Read the model definition and answer for the solid it produces. Units are mm, in the model's axes. A direction names the side the tool comes from. Coordinates: 2 decimals unless noted, no trailing zeros. Loops run counter-clockwise (first coordinate to the right, second up) from the corner with the lowest first, then second, coordinate; pieces in that order, holes last. Notation, with made-up numbers: M -37,46 L -8,46 A25 ccw -8,58 Z; hole C 29,71.5 d10. An arc over 180 degrees is marked long. One line per item, written item: value. Start each with the question number.
```python
from build123d import *

# Parameters (mm, degrees)
SKETCH1_W           = 93.8
SKETCH1_H           = 32.4
BOSS_EXTRUDE1_DEPTH = 2
SKETCH3_W           = 93.8
SKETCH3_H           = 64.8
SKETCH3_W_2         = 91.4
SKETCH3_H_2         = 62.4
SKETCH3_W_3         = 86.6
SKETCH3_H_3         = 57.6
SKETCH3_W_4         = 83.8
SKETCH3_H_4         = 54.8
BOSS_EXTRUDE2_DEPTH = 4
FILLET6_R           = 2
FILLET8_START       = -66
FILLET8_DEPTH       = 67
FILLET9_R           = 2
FILLET10_R          = 2


with BuildPart() as part:
    # Sketch1 → Boss-Extrude1 (new body)
    with BuildSketch(Plane(origin=(0, 0, 0), x_dir=(1, 0, 0), z_dir=(0, 1, 0))):
        with Locations((46.9, 48.6)):
            Rectangle(SKETCH1_W, SKETCH1_H)
        Polygon((93.8, 32.4), (0, 32.4), (0, 0), (42.9, 0), (50.9, 0), (93.8, 0), align=None)
    extrude(amount=BOSS_EXTRUDE1_DEPTH)

    # Sketch3 → Boss-Extrude2 (add)
    # profile 1 of 2: a face of its own
    with BuildSketch(Plane.XZ):
        with Locations((46.9, -32.4)):
            Rectangle(SKETCH3_W, SKETCH3_H)
        with Locations((46.9, -32.4)):
            Rectangle(SKETCH3_W_2, SKETCH3_H_2, mode=Mode.SUBTRACT)
    # profile 2 of 2: a face of its own
    with BuildSketch(Plane.XZ):
        with Locations((46.9, -32.4)):
            Rectangle(SKETCH3_W_3, SKETCH3_H_3)
        with Locations((46.9, -32.4)):
            Rectangle(SKETCH3_W_4, SKETCH3_H_4, mode=Mode.SUBTRACT)
    extrude(amount=BOSS_EXTRUDE2_DEPTH)

    # Fillet6
    fillet6_edges = [part.edges().sort_by_distance(p)[0] for p in [
        (0, -1, -64.8),
        (93.8, -1, -64.8),
        (93.8, -1, 0),
        (0, -1, 0),
    ]]
    fillet(fillet6_edges, radius=FILLET6_R)

    # Fillet8: read off the stored shape, not the designer's step
    # Fillet8 outline → Fillet8 (cut)
    with BuildSketch(Plane.XY.offset(FILLET8_START)):
        with BuildLine():
            add(Edge.make_bspline(
                [(0, -1), (0, 2), (4, 2)],
                knots=[0, 0, 0, 1, 1, 1], degree=2, weights=[1, 0.707106781, 1]))
            Line((4, 2), (0, 2))
            Line((0, 2), (0, -1))
        make_face()
        with BuildLine():
            add(Edge.make_bspline(
                [(93.8, -1), (93.8, 2), (89.8, 2)],
                knots=[0, 0, 0, 1, 1, 1], degree=2, weights=[1, 0.707106781, 1]))
            Line((93.8, -1), (93.8, 2))
            Line((93.8, 2), (89.8, 2))
        make_face()
    extrude(amount=FILLET8_DEPTH, mode=Mode.SUBTRACT)

    # Fillet9
    fillet9_edges = [part.edges().sort_by_distance(p)[0] for p in [
        (5, 0, -32.4),
        (46.9, 0, -5),
        (88.8, 0, -32.4),
        (46.9, 0, -59.8),
    ]]
    fillet(fillet9_edges, radius=FILLET9_R)

    # Fillet10
    fillet10_edges = [part.edges().sort_by_distance(p)[0] for p in [
        (92.6, -2, -1.2),
    ]]
    fillet(fillet10_edges, radius=FILLET10_R)


solid = part.part
```
1) A flat-ended cylindrical pin translates along its axis: pin 1 (18.5 mm diameter, centred on x = 69, z = -23, fed in from -Y). Find the tip coordinate at first contact, or state that the pin passes through.
2) A tool of negligible diameter and unlimited length cuts with its end or side. For faces 1 (the face through (47, -4, -1)), 2 (the face through (92.6, -2, -34)), from which of +Z, -Z, +X, -X, +Y, -Y can it reach the whole face along a straight path? Write none if from no direction.
3) Section A-A (x = 35) is taken. Determine the outline of the cut face in (y, z).
4) Consider line 1 along Z through (x, y) = (56.5, -2.75); line 2 along X through (y, z) = (-2.25, -29); line 3 along X through (y, z) = (-0.5, -55). Determine where each line is inside the solid, lowest interval first.
5) For a pull along Z with two mould halves and no side action, classify faces 3 (the face through (47.49, -0.6, -59.23)), 4 (the face through (93.23, -1.78, -0.6)), 5 (the face through (0.57, -1.86, -64.2)) as released by +Z, released by -Z, zero draft, split by the parting line, or undercut.
Results found:
1. pin 1: stops at y = 0
2. face 1: +Z, -Z, +X, -X, -Y
2. face 2: -Y
3. outline: M -4,-64.8 L 2,-64.8 L 2,0 L -4,0 L -4,-1.2 L 0,-1.2 L 0,-3.6 L -4,-3.6 L -4,-5 L -2,-5 A2 cw 0,-7 L 0,-57.8 A2 cw -2,-59.8 L -4,-59.8 L -4,-61.2 L 0,-61.2 L 0,-63.6 L -4,-63.6 Z
4. line 1: z = -64.8 to -63.6, -61.2 to -59.8, -5 to -3.6, -1.2 to 0
4. line 2: x = 0 to 1.2, 3.6 to 5, 88.8 to 90.2, 92.6 to 93.8
4. line 3: x = 0.06 to 1.2, 3.6 to 5.68, 88.12 to 90.2, 92.6 to 93.74
5. face 3: undercut
5. face 4: released by +Z
5. face 5: released by -Z
